CAD build for the part. Positions are in the model's coordinates, mm. A direction names the side the tool comes from. Round coordinates to 2 decimals unless told otherwise and drop trailing zeros. Order: outer loops, then holes, each group sorted by start corner. A loop starts at its lowest first (then second) coordinate and runs counter-clockwise, first axis right, second up. Notation, with made-up numbers: (70, -38.5) -> (104, -38.5) arc R11 cw to (104, -31.5) -> close; hole circle Ø1 at (8, 42.5). An arc over 180 degrees is marked (long way). Return JSON: item names as keys, results as strings. Group by question number.
Q1. Probe line 1 along X through (y, z) = (1, 6); line 2 along Y through (x, z) = (30.5, -12.5); line 3 along X through (y, z) = (8, -19). List the from-to ranges inside material, lowest first.
Q2. Which spindle directions (+Z, -Z, +X, -X, +Y, -Y) get a long thin tool onto all of the face, cutting with end or side? Do faces 1 (the cylindrical face through (27.53, -6.76, 21.46)), 2 (the flat face through (20, -0.1, -3.3)). Say none if no direction does.
Q3. Cut at A-A (x = 17.5). Write the cut outline in (y, z), then the cut area to 3 significant figures.
Q4. Flat gauge pins, fed straight in: pin 1 (4 mm diameter, centred on x = 28, z = -10.5, fed in from -Y); pin 2 (12 mm diameter, centred on x = 19.5, z = 4, fed in from -Y); pin 3 (12 mm diameter, centred on x = 21, z = 11, fed in from -Y). Where does each tip first touch, or does it go through?
from build123d import *

# Parameters (mm, degrees)
FILLET_1_R = 2


with BuildPart() as part:
    # Эскиз1 → Повернуть1 (revolve)
    with BuildSketch(Plane.XY, mode=Mode.PRIVATE) as revolve_1_sk:
        Polygon((0, 0), (0, 3), (20, 3), (20, 7.57179677), (24, 22.5), (31, 22.5), (35, 7.57179677), (35, 0), (26, 0), align=None)
    revolve(revolve_1_sk.sketch.rotate(Axis((0, 0, 0), (1, 0, 0)), 90), axis=Axis((0, 0, 0), (1, 0, 0)))

    # Скругление1
    fillet_1_edges = [part.edges().sort_by_distance(p)[0] for p in [
        (31, 0, -22.5),
        (24, 0, -22.5),
    ]]
    fillet(fillet_1_edges, radius=FILLET_1_R)


solid = part.part
Solution:
{
 "1": {"line 1": "x = 20 to 35", "line 2": "y = -18.36 to 18.36", "line 3": "x = 23.5 to 31.5"},
 "2": {"face 1": "+X, -X", "face 2": "-X"},
 "3": {"outline": "circle Ø6 at (0, 0)", "area": "28.3 mm²"},
 "4": {"pin 1": "stops at y = -20.83", "pin 2": "stops at y = -22.38", "pin 3": "stops at y = -21.46"}
}
